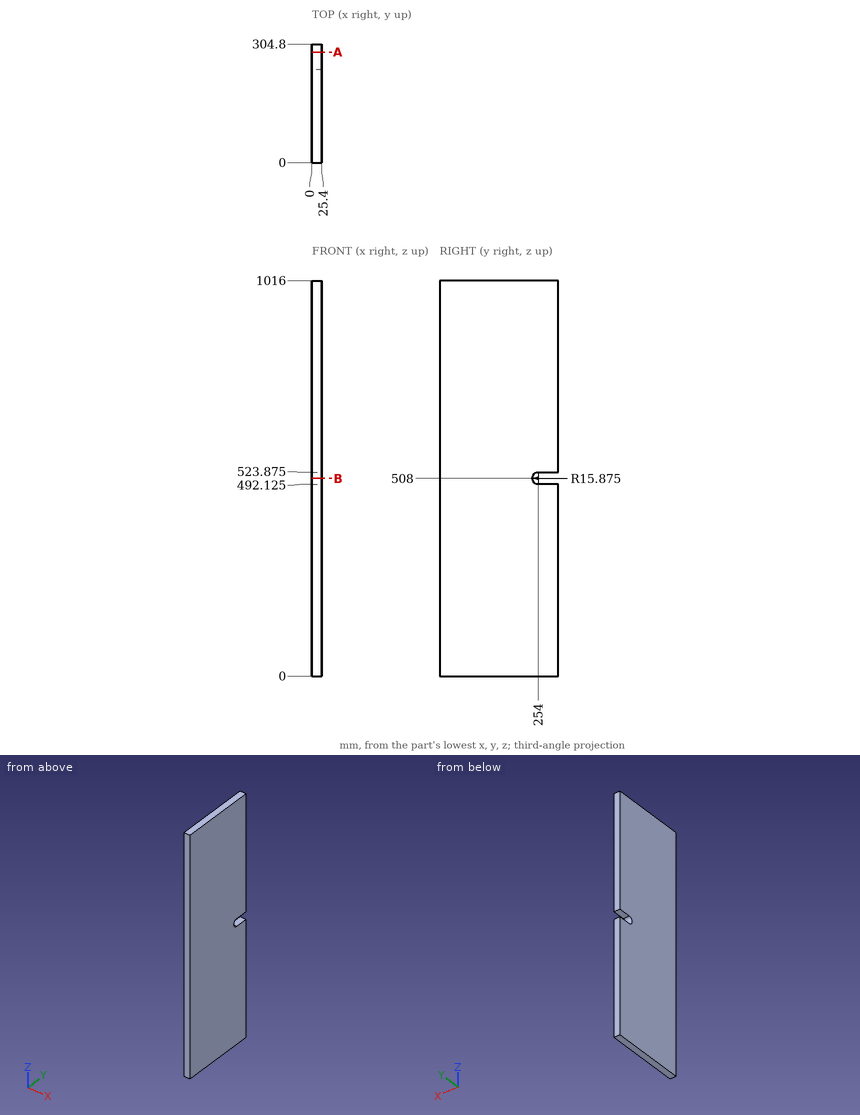
Could you check a few things on this drawing? It's one solid part, dimensions in mm from its lowest x, y, z. Round coordinates to 2 decimals unless told otherwise and drop trailing zeros. Loops run counter-clockwise (first coordinate to the right, second up) from the corner with the lowest first, then second, coordinate; pieces in that order, holes last.
Q1. For P1, Ø6, axis at x = 3, y = 154, coming from the -Z side, with a flat end and sliding along its axis, tell me the tip position at first contact or that it passes through.
Q2. I want a section at A-A (y = 284). Write out the boundary of the cut face in (x, z) (3 decimals), and give its area (3 significant figures).
Q3. Please list where these lines run through material, in increasing order: L1, parallel to Z at x = 16.5, y = 270 (3 decimals); L2, parallel to Z at x = 15.25, y = 252; L3, parallel to Y at x = 20.75, z = 501.
Q4. I want a section at B-B (z = 508). Write out the boundary of the cut face in (x, y) (3 decimals).
Answer below:
1. P1: stops at z = 0
2. outline: (0, 0) - (25.4, 0) - (25.4, 492.125) - (0, 492.125) - close; (0, 523.875) - (25.4, 523.875) - (25.4, 1016) - (0, 1016) - close
2. area: 25,000 mm2
3. L1: z = 0 to 492.125, 523.875 to 1016
3. L2: z = 0 to 492.25, 523.75 to 1016
3. L3: y = 0 to 239.75
4. outline: (0, 0) - (25.4, 0) - (25.4, 238.125) - (0, 238.125) - close
